from build123d import *

# Parameters (mm, degrees)
BOSS_EXTRUDE2_DEPTH     = 19.5
SKETCH4_W               = 27
SKETCH4_H               = 23.2
CUT_EXTRUDE2_DEPTH      = 15.1
CUT_EXTRUDE2_DEPTH_BACK = 15.1
CUT_EXTRUDE4_DEPTH      = 3
SKETCH5_R               = 1.6
CUT_EXTRUDE5_DEPTH      = 14.1
CUT_EXTRUDE5_DEPTH_BACK = 14.1


with BuildPart() as part:
    # Sketch2 → Boss-Extrude2 (new body, symmetric)
    with BuildSketch(Plane.XY):
        with BuildLine():
            Line((-14.1, -13.1), (14.1, -13.1))
            Line((14.1, -13.1), (14.1, -1))
            ThreePointArc((14.1, -1), (0, 13.1), (-14.1, -1))
            Line((-14.1, -1), (-14.1, -13.1))
        make_face()
        with BuildLine():
            Line((6.25, 9.360863864), (6.25, -10.1))
            Line((6.25, -10.1), (7.974960815, -10.1))
            ThreePointArc((7.974960815, -10.1), (12.052745875, 0.06832433), (6.25, 9.360863864))
        make_face(mode=Mode.SUBTRACT)
        with BuildLine():
            Line((-6.25, 9.360863864), (-6.25, -10.1))
            Line((-6.25, -10.1), (-7.974960815, -10.1))
            ThreePointArc((-7.974960815, -10.1), (-12.052745875, 0.06832433), (-6.25, 9.360863864))
        make_face(mode=Mode.SUBTRACT)
        with BuildLine():
            Line((2.061552813, -5), (-2.061552813, -5))
            ThreePointArc((-2.061552813, -5), (0, 3.5), (2.061552813, -5))
        make_face(mode=Mode.SUBTRACT)
    extrude(amount=BOSS_EXTRUDE2_DEPTH, both=True)

    # Sketch4 → Cut-Extrude2 (cut, two sides)
    with BuildSketch(Plane(origin=(0, 0, 0), x_dir=(0, 0, -1), z_dir=(1, 0, 0))) as cut_extrude2_sk:
        with Locations((0, 1.5)):
            Rectangle(SKETCH4_W, SKETCH4_H)
    extrude(amount=CUT_EXTRUDE2_DEPTH, mode=Mode.SUBTRACT)
    extrude(cut_extrude2_sk.sketch, amount=-CUT_EXTRUDE2_DEPTH_BACK, mode=Mode.SUBTRACT)

    # Sketch3 → Cut-Extrude4 (cut)
    with BuildSketch(Plane.XY.offset(19.5)):
        with BuildLine():
            Line((-12.6, -1), (-12.6, -13.1))
            Line((-12.6, -13.1), (12.6, -13.1))
            Line((12.6, -13.1), (12.6, -1))
            ThreePointArc((12.6, -1), (0, 11.6), (-12.6, -1))
        make_face()
    cut_extrude4 = extrude(amount=-CUT_EXTRUDE4_DEPTH, mode=Mode.SUBTRACT)

    # Sketch5 → Cut-Extrude5 (cut, two sides)
    with BuildSketch(Plane(origin=(0, 0, 0), x_dir=(1, 0, 0), z_dir=(0, 1, 0))) as cut_extrude5_sk:
        with Locations((7.5, 0)):
            Circle(SKETCH5_R)
        with Locations((-7.5, 0)):
            Circle(SKETCH5_R)
    extrude(amount=CUT_EXTRUDE5_DEPTH, mode=Mode.SUBTRACT)
    extrude(cut_extrude5_sk.sketch, amount=-CUT_EXTRUDE5_DEPTH_BACK, mode=Mode.SUBTRACT)

    # Mirror2: Cut-Extrude4 across plane
    add(cut_extrude4.mirror(Plane.XY), mode=Mode.SUBTRACT)


solid = part.part
Work out the finished part from the listing and answer in its coordinate system (mm). A direction names the side the tool comes from. Give positions to 0.01 mm unless a question says otherwise; leave off trailing zeros. Loops run counter-clockwise (first coordinate to the right, second up) from the corner with the lowest first, then second, coordinate; pieces in that order, holes last. Notation, with made-up numbers: (58, -29.5) -> (106, -29.5) arc R29 ccw to (106, 4.5) -> close; hole circle Ø6 at (10.25, -33). An arc over 180 degrees is marked (long way). Use a Markdown table: item, result. Add a question column.
1. Flat-ended cylindrical pins translate along their axes: pin 1 Ø14.5 at (x, y) = (0, -1) entering from +Z; pin 2 Ø6 at (x, z) = (8, 5.5) entering from +Y; pin 3 Ø8 at (x, y) = (-4, -4) entering from -Z. Find the tip coordinate at first contact, or state that the pin passes through.
2. Determine the mould class of faces 1 (the cylindrical face through (12.066, -0.09, -14.979)), 2 (the flat face through (12.6, -7, 18)), 3 (the cylindrical face through (0.31, 13.097, -16.458)) for opening direction Y: released by +Y, released by -Y, zero draft, split by the parting line, or undercut.
3. Section C-C on x = 7.5 is taken. Determine the outline of the cut face in (y, z), and give its area (3 significant figures).
4. Section A-A on z = 0 is taken. Determine the outline of the cut face in (x, y).
5. For faces 4 (the flat face through (6.25, 0, -15)), 5 (the cylindrical face through (0.277, 11.597, 18.021)), 6 (the flat face through (0, 4, -13.5)), determine the directions among +Z, -Z, +X, -X, +Y, -Y from which every point of the face is accessible in a straight line to the end or side of a thin tool.
6. Section B-B on x = 0 is taken. Determine the outline of the cut face in (y, z).
7. Section D-D on y = 4.75 is taken. State how many separate pieces and enclosed holes the cut face has, and give its area (3 significant figures).
8. Find the intervals of material crossed by probe 1 along X at (y, z) = (-10.7, 0); probe 2 along Z at (x, y) = (-7.5, -11.8); probe 3 along Z at (x, y) = (3.5, -6), in increasing order.
Results below:
| question | item | result |
|---|---|---|
| 1 | pin 1 | stops at z = 16.5 |
| 1 | pin 2 | stops at y = -10.1 |
| 1 | pin 3 | stops at z = -16.5 |
| 2 | face 1 | undercut |
| 2 | face 2 | zero draft |
| 2 | face 3 | released by +Y |
| 3 | outline | (-13.1, -16.5) -> (-10.1, -16.5) -> (-10.1, -1.6) -> (-13.1, -1.6) -> close; (-13.1, 1.6) -> (-10.1, 1.6) -> (-10.1, 16.5) -> (-13.1, 16.5) -> close; (8.5, -16.5) -> (9.12, -16.5) -> (9.12, -19.5) -> (10.94, -19.5) -> (10.94, -13.5) -> (8.5, -13.5) -> close; (8.5, 13.5) -> (10.94, 13.5) -> (10.94, 19.5) -> (9.12, 19.5) -> (9.12, 16.5) -> (8.5, 16.5) -> close |
| 3 | area | 115 mm^2 |
| 4 | outline | (-14.1, -13.1) -> (-9.1, -13.1) -> (-9.1, -10.1) -> (-14.1, -10.1) -> close; (-5.9, -13.1) -> (5.9, -13.1) -> (5.9, -10.1) -> (-5.9, -10.1) -> close; (9.1, -13.1) -> (14.1, -13.1) -> (14.1, -10.1) -> (9.1, -10.1) -> close |
| 5 | face 4 | +Z, -Z |
| 5 | face 5 | +Z, -Y |
| 5 | face 6 | +X, -X, +Y |
| 6 | outline | (-13.1, -16.5) -> (-5, -16.5) -> (-5, -13.5) -> (-10.1, -13.5) -> (-10.1, 13.5) -> (-5, 13.5) -> (-5, 16.5) -> (-13.1, 16.5) -> close; (3.5, -16.5) -> (11.6, -16.5) -> (11.6, -19.5) -> (13.1, -19.5) -> (13.1, -13.5) -> (3.5, -13.5) -> close; (3.5, 13.5) -> (13.1, 13.5) -> (13.1, 19.5) -> (11.6, 19.5) -> (11.6, 16.5) -> (3.5, 16.5) -> close |
| 7 | separate pieces | 6 |
| 7 | enclosed holes | 0 |
| 7 | area | 122 mm^2 |
| 8 | probe 1 | x = -14.1 to -9.1, -5.9 to 5.9, 9.1 to 14.1 |
| 8 | probe 2 | z = -16.5 to -1.6, 1.6 to 16.5 |
| 8 | probe 3 | z = -16.5 to -13.5, 13.5 to 16.5 |
